from build123d import *

# Parameters (mm, degrees)
BOSS_EXTRUDE1_DEPTH     = 20
CUT_EXTRUDE1_REACH      = 75.485
CUT_EXTRUDE1_END_RADIUS = 50
SKETCH3_R               = 2.75
CUT_EXTRUDE2_REACH      = 70.602
CUT_EXTRUDE2_END_RADIUS = 50
SKETCH4_R               = 4.5
FILLET1_R               = 10
FILLET2_R               = 3


with BuildPart() as part:
    # Sketch2 → Boss-Extrude1 (new body)
    with BuildSketch(Plane.XY):
        with BuildLine():
            Line((0, 0), (-45.315389352, 21.130913087))
            ThreePointArc((-45.315389352, 21.130913087), (-42.169572291, -26.864980417), (0, -50))
            Line((0, -50), (0, 0))
        make_face()
    extrude(amount=BOSS_EXTRUDE1_DEPTH)

    # Cut-Extrude1: up to this cylinder (the profile starts inside it)
    cut_extrude1_end = Plane(origin=(0, 0, 10), z_dir=(0, 0, -1)) * Cylinder(CUT_EXTRUDE1_END_RADIUS, 251.97, mode=Mode.PRIVATE)
    # Sketch3 → Cut-Extrude1 (cut, up to the surface)
    with BuildSketch(Plane(origin=(0, 0, 0), x_dir=(0, 0, -1), z_dir=(1, 0, 0)), mode=Mode.PRIVATE) as cut_extrude1_sk1:
        with Locations(Location((-10, -35, 0), (0, 0, 90))):
            Circle(SKETCH3_R)
    cut_extrude1_tool1 = extrude(cut_extrude1_sk1.sketch, amount=-CUT_EXTRUDE1_REACH, mode=Mode.PRIVATE) & cut_extrude1_end
    add(cut_extrude1_tool1.solids().sort_by_distance((0, -35, 10))[0], mode=Mode.SUBTRACT)
    # Sketch3 → Cut-Extrude1 (cut, up to the surface)
    with BuildSketch(Plane(origin=(0, 0, 0), x_dir=(0, 0, -1), z_dir=(1, 0, 0)), mode=Mode.PRIVATE) as cut_extrude1_sk2:
        with Locations(Location((-10, -15, 0), (0, 0, 90))):
            Circle(SKETCH3_R)
    cut_extrude1_tool2 = extrude(cut_extrude1_sk2.sketch, amount=-CUT_EXTRUDE1_REACH, mode=Mode.PRIVATE) & cut_extrude1_end
    add(cut_extrude1_tool2.solids().sort_by_distance((0, -15, 10))[0], mode=Mode.SUBTRACT)

    # Cut-Extrude2: up to this cylinder (the profile starts inside it)
    cut_extrude2_end = Plane(origin=(0, 0, 10), z_dir=(0, 0, -1)) * Cylinder(CUT_EXTRUDE2_END_RADIUS, 242.204, mode=Mode.PRIVATE)
    # Sketch4 → Cut-Extrude2 (cut, up to the surface)
    with BuildSketch(Plane(origin=(-7.5, 0, 0), x_dir=(0, 0, -1), z_dir=(1, 0, 0)), mode=Mode.PRIVATE) as cut_extrude2_sk1:
        with Locations(Location((-10, -15, 0), (0, 0, 90))):
            Circle(SKETCH4_R)
    cut_extrude2_tool1 = extrude(cut_extrude2_sk1.sketch, amount=-CUT_EXTRUDE2_REACH, mode=Mode.PRIVATE) & cut_extrude2_end
    add(cut_extrude2_tool1.solids().sort_by_distance((-7.5, -15, 10))[0], mode=Mode.SUBTRACT)
    # Sketch4 → Cut-Extrude2 (cut, up to the surface)
    with BuildSketch(Plane(origin=(-7.5, 0, 0), x_dir=(0, 0, -1), z_dir=(1, 0, 0)), mode=Mode.PRIVATE) as cut_extrude2_sk2:
        with Locations(Location((-10, -35, 0), (0, 0, 90))):
            Circle(SKETCH4_R)
    cut_extrude2_tool2 = extrude(cut_extrude2_sk2.sketch, amount=-CUT_EXTRUDE2_REACH, mode=Mode.PRIVATE) & cut_extrude2_end
    add(cut_extrude2_tool2.solids().sort_by_distance((-7.5, -35, 10))[0], mode=Mode.SUBTRACT)

    # Fillet1
    # the kernel refuses this fillet: 10 mm, written as the material it takes off along each edge
    with BuildSketch(Plane(origin=(0, 0, 20), x_dir=(-0.5924817254083071, 0.8055838907632124, 0), z_dir=(0.8055838907632124, 0.5924817254083071, 0))) as fillet1_piece_1:
        with BuildLine():
            CenterArc((50 - FILLET1_R, -FILLET1_R), FILLET1_R, 0, 90)
            Line((50 - FILLET1_R, 0), (50, 0))
            Line((50, 0), (50, -FILLET1_R))
        make_face()
    revolve(axis=Axis((0, 0, 20), (0, 0, 1)), revolution_arc=172.333365089, mode=Mode.SUBTRACT)

    # Fillet2
    fillet2_edges = [part.edges().sort_by_distance(p)[0] for p in [
        (0, -20, 20),
        (0, -50, 5),
        (0, -47.071067812, 17.071067812),
        (-45.315389352, 21.130913087, 5),
        (-42.660875302, 19.893092857, 17.071067812),
        (-18.126155741, 8.452365235, 20),
    ]]
    fillet(fillet2_edges, radius=FILLET2_R)


solid = part.part
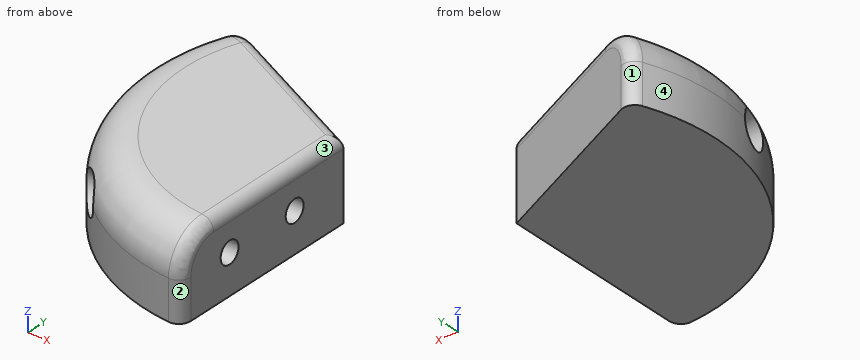
Build history of the part. All positions in model axes, mm. Face numbers are marked on the shaded views. Round coordinates to 2 decimals unless told otherwise and drop trailing zeros. Answer as a JSON object with one key per item and string values. Group by question number.
(1) Cut at A-A (x = -17). Give the number of separate pieces and of enclosed holes in the cut face, and give its area (3 significant figures).
(2) Mould opens along Y. For the marked faces 1, 2, 3 and 4 say: pulls with the +Y half, pulls with the -Y half, needs draft (parallel to the pull), parting line crosses it, or undercut.
(3) Flat gauge pins, fed straight in: pin 1 (10.5 mm diameter, centred on y = -15, z = 10, fed in from -X); pin 2 (2 mm diameter, centred on x = -7.5, z = 17, fed in from -Y); pin 3 (8 mm diameter, centred on y = -35, z = 10, fed in from +X); pin 4 (7 mm diameter, centred on y = -35, z = 10, fed in from -X). Where does each tip first touch, or does it go through?
(4) Drill centre lines: L1, parallel to Z at x = -4, y = -15; L2, parallel to Y at x = -28.5, z = 10; L3, parallel to Y at x = -24, z = 10. Where is each one in solid material? Low to high.
Responses:
{
 "1": {"separate pieces": "1", "enclosed holes": "2", "area": "947 mm2"},
 "2": {"face 1": "pulls with the +Y half", "face 2": "pulls with the -Y half", "face 3": "needs draft", "face 4": "parting line crosses it"},
 "3": {"pin 1": "stops at x = -49.04", "pin 2": "stops at y = -47.43", "pin 3": "stops at x = 0", "pin 4": "stops at x = -7.5"},
 "4": {"L1": "z = 0 to 7.25, 12.75 to 20", "L2": "y = -41.08 to -39.5, -30.5 to -19.5, -10.5 to 13.29", "L3": "y = -43.86 to -39.5, -30.5 to -19.5, -10.5 to 11.19"}
}
